Answer from the drawing. Dimensions are ordinates in mm from the lowest x, y and z of the part. Coordinates: 2 decimals unless noted, no trailing zeros. Order: outer loops, then holes, each group sorted by start corner. A loop starts at its lowest first (then second) coordinate and runs counter-clockwise, first axis right, second up. Notation, with made-up numbers: (10, -27) -> (27, -27) arc R5 cw to (27, -21) -> close; hole circle Ø10 at (0.5, 22). An arc over 180 degrees is marked (long way). Answer as a JSON object with one key per item and string values. Group by question number.
1) Consider L1, parallel to Z at x = 5, y = 3.85; L2, parallel to Z at x = 71, y = 4.55; L3, parallel to X at y = 0.55, z = 43. Determine where each line is inside the solid, lowest interval first.
2) Given pin 1 (1.5 mm diameter, centred on y = 1, z = 29.5, fed in from +X); pin 2 (5.5 mm diameter, centred on x = 5, z = 51, fed in from -Y); pin 3 (1.8 mm diameter, centred on x = 5, z = 51, fed in from +Y); pin 4 (2 mm diameter, centred on x = 32.5, y = 2.5, fed in from +Z), each flat-ended and moving along its own axis, determine where each tip first touches the part or whether it passes through.
3) Section C-C on y = 4.2 is taken. Determine the outline of the cut face in (x, z), and give its area (3 significant figures).
4) Section A-A on z = 5 is taken. Determine the outline of the cut face in (x, y).
5) Section B-B on x = 5 is taken. Determine the outline of the cut face in (y, z), and give its area (3 significant figures).
6) Section D-D on x = 71 is taken. Determine the outline of the cut face in (y, z), and give its area (3 significant figures).
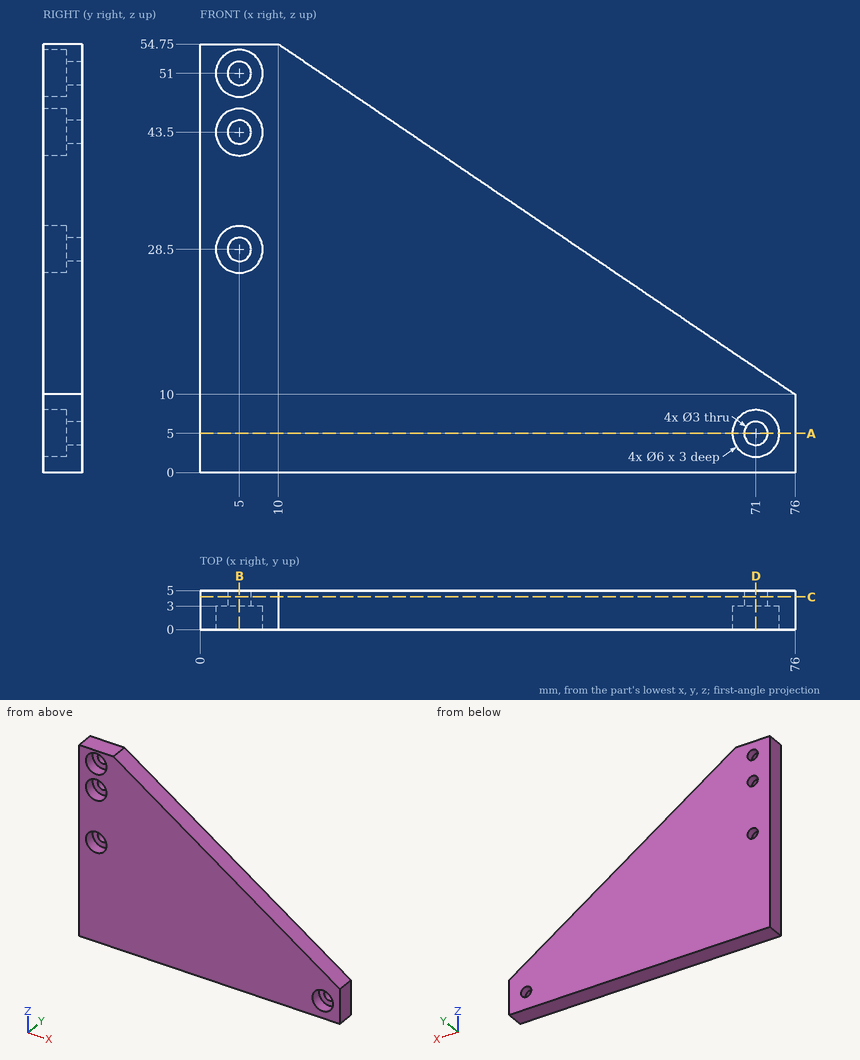
Worked answers:
{
 "1": {"L1": "z = 0 to 27, 30 to 42, 45 to 49.5, 52.5 to 54.75", "L2": "z = 0 to 3.5, 6.5 to 13.39", "L3": "x = 0 to 2.04, 7.96 to 27.33"},
 "2": {"pin 1": "stops at x = 48.35", "pin 2": "stops at y = 3", "pin 3": "passes through", "pin 4": "stops at z = 40.17"},
 "3": {"outline": "(0, 0) -> (76, 0) -> (76, 10) -> (10, 54.75) -> (0, 54.75) -> close; hole circle Ø3 at (5, 28.5); hole circle Ø3 at (5, 43.5); hole circle Ø3 at (5, 51); hole circle Ø3 at (71, 5)", "area": "2,660 mm²"},
 "4": {"outline": "(0, 0) -> (68, 0) -> (68, 3) -> (69.5, 3) -> (69.5, 5) -> (0, 5) -> close; (72.5, 3) -> (74, 3) -> (74, 0) -> (76, 0) -> (76, 5) -> (72.5, 5) -> close"},
 "5": {"outline": "(0, 0) -> (5, 0) -> (5, 27) -> (3, 27) -> (3, 25.5) -> (0, 25.5) -> close; (0, 31.5) -> (3, 31.5) -> (3, 30) -> (5, 30) -> (5, 42) -> (3, 42) -> (3, 40.5) -> (0, 40.5) -> close; (0, 46.5) -> (3, 46.5) -> (3, 45) -> (5, 45) -> (5, 49.5) -> (3, 49.5) -> (3, 48) -> (0, 48) -> close; (0, 54) -> (3, 54) -> (3, 52.5) -> (5, 52.5) -> (5, 54.75) -> (0, 54.75) -> close", "area": "202 mm²"},
 "6": {"outline": "(0, 0) -> (5, 0) -> (5, 3.5) -> (3, 3.5) -> (3, 2) -> (0, 2) -> close; (0, 8) -> (3, 8) -> (3, 6.5) -> (5, 6.5) -> (5, 13.39) -> (0, 13.39) -> close", "area": "43.0 mm²"}
}
